```python
from build123d import *

# Parameters (mm, degrees)
ESBO_O1_W                = 126
ESBO_O1_H                = 74
ESBO_O1_W_2              = 120
ESBO_O1_H_2              = 68
RESSALTO_EXTRUS_O1_DEPTH = 60
ESBO_O2_W                = 126
ESBO_O2_H                = 74
ESBO_O2_R                = 2
RESSALTO_EXTRUS_O2_DEPTH = 2
ESBO_O3_W                = 25
ESBO_O3_H                = 25
ESBO_O3_W_2              = 14
ESBO_O3_H_2              = 16
ESBO_O3_W_3              = 10
ESBO_O3_H_3              = 30
CORTE_EXTRUS_O1_DEPTH    = 10
ESBO_O6_W                = 8
ESBO_O6_H                = 40
CORTE_EXTRUS_O2_DEPTH    = 115.214710086
ESBO_O7_W                = 10
ESBO_O7_H                = 30
CORTE_EXTRUS_O3_DEPTH    = 12


with BuildPart() as part:
    # Esboço1 → Ressalto-extrusão1 (new body)
    with BuildSketch(Plane.XY):
        Rectangle(ESBO_O1_W, ESBO_O1_H)
        Rectangle(ESBO_O1_W_2, ESBO_O1_H_2, mode=Mode.SUBTRACT)
    extrude(amount=RESSALTO_EXTRUS_O1_DEPTH)

    # Esboço2 → Ressalto-extrusão2 (add)
    with BuildSketch(Plane(origin=(0, 0, 0), x_dir=(-1, 0, 0), z_dir=(0, 0, -1))):
        Rectangle(ESBO_O2_W, ESBO_O2_H)
        with Locations((-54, -28)):
            Circle(ESBO_O2_R, mode=Mode.SUBTRACT)
        with Locations((54, -28)):
            Circle(ESBO_O2_R, mode=Mode.SUBTRACT)
        with Locations((54, 28)):
            Circle(ESBO_O2_R, mode=Mode.SUBTRACT)
        with Locations((-54, 28)):
            Circle(ESBO_O2_R, mode=Mode.SUBTRACT)
    extrude(amount=RESSALTO_EXTRUS_O2_DEPTH)

    # Esboço3 → Corte-extrusão1 (cut)
    with BuildSketch(Plane(origin=(63, 0, 0), x_dir=(0, 0, -1), z_dir=(1, 0, 0))):
        with Locations((-23.5, 19.5)):
            Rectangle(ESBO_O3_W, ESBO_O3_H)
        with Locations((-7, -15.5)):
            Rectangle(ESBO_O3_W_2, ESBO_O3_H_2)
        with Locations((-45, 0)):
            Rectangle(ESBO_O3_W_3, ESBO_O3_H_3)
    extrude(amount=-CORTE_EXTRUS_O1_DEPTH, mode=Mode.SUBTRACT)

    # Esboço6 → Corte-extrusão2 (cut, through all)
    with BuildSketch(Plane.XZ.offset(37)):
        with Locations((-49, 28)):
            Rectangle(ESBO_O6_W, ESBO_O6_H)
        with Locations((-36, 28)):
            Rectangle(ESBO_O6_W, ESBO_O6_H)
        with Locations((-23, 28)):
            Rectangle(ESBO_O6_W, ESBO_O6_H)
        with Locations((-10, 28)):
            Rectangle(ESBO_O6_W, ESBO_O6_H)
        with Locations((3, 28)):
            Rectangle(ESBO_O6_W, ESBO_O6_H)
        with Locations((16, 28)):
            Rectangle(ESBO_O6_W, ESBO_O6_H)
        with Locations((29, 28)):
            Rectangle(ESBO_O6_W, ESBO_O6_H)
        with Locations((42, 28)):
            Rectangle(ESBO_O6_W, ESBO_O6_H)
    extrude(amount=-CORTE_EXTRUS_O2_DEPTH, mode=Mode.SUBTRACT)

    # Esboço7 → Corte-extrusão3 (cut)
    with BuildSketch(Plane.ZY.offset(63)):
        with Locations((43, 0)):
            Rectangle(ESBO_O7_W, ESBO_O7_H)
        with Locations((23, 0)):
            Rectangle(ESBO_O7_W, ESBO_O7_H)
    extrude(amount=-CORTE_EXTRUS_O3_DEPTH, mode=Mode.SUBTRACT)


solid = part.part
```
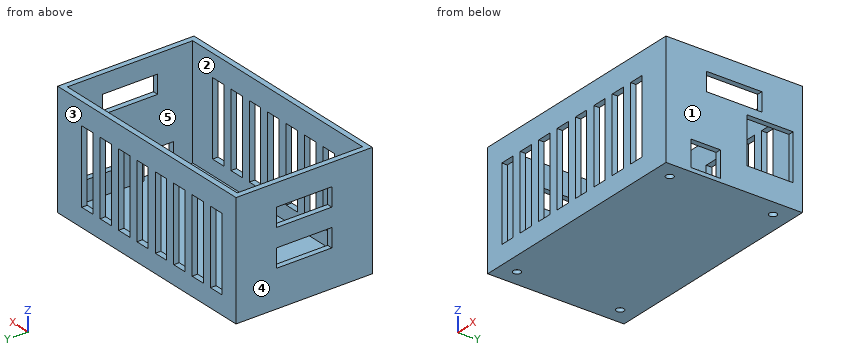
Can you work these out from the model? Positions are in its coordinate system, mm. Face numbers are marked on the shaded views. A direction names the side the tool comes from. Coordinates: 2 decimals unless noted, no trailing zeros. Loops run counter-clockwise (first coordinate to the right, second up) from the corner with the lowest first, then second, coordinate; pieces in that order, holes last. Notation, with made-up numbers: (-37, 39) -> (-17, 39) arc R4 cw to (-17, 43) -> close; hole circle Ø9 at (82.25, -35). An arc over 180 degrees is marked (long way). Put each result on its own line as item: value. Start each with the question number.
Q1. I want a section at D-D (y = -18.5). Write out the boundary of the cut face in (x, z), plus the area to 3 significant figures.
Q2. Thinking about a two-plate mould opening in Y: for the marked faces 3, 4 and 5, which applies, pulls with the +Y half, pulls with the -Y half, needs draft (parallel to the pull), parting line crosses it, or undercut?
Q3. I want a section at A-A (y = 28). Write out the boundary of the cut face in (x, z), plus the area to 3 significant figures.
Q4. I want a section at C-C (x = -22). Write out the boundary of the cut face in (y, z), plus the area to 3 significant figures.
Q5. If I drill on line 1 (Y direction, x = -48.5, z = 3); line 2 (X direction, y = -10.5, z = 51.5); line 3 (Y direction, x = -54, z = -1.15), over which ranges is the centre line in solid material (lowest first)? Write a range as [from, to].
Q6. I want a section at B-B (z = 55). Write out the boundary of the cut face in (x, y), plus the area to 3 significant figures.
Q7. I'm going to push flat-ended pins straight in: P1, Ø12, axis at x = -20, y = -22, coming from the +Z side; P2, Ø8, axis at y = -9, z = 26.5, coming from the -X side. Where does each tip first touch, or does it pass through?
Q8. For the marked faces 1 and 2, which set-ups out of +Z, -Z, +X, -X, +Y, -Y let a thin tool reach every point of the face, with its end or its side?
Taken from the geometry:
1. outline: (-63, -2) -> (63, -2) -> (63, 0) -> (-60, 0) -> (-60, 60) -> (-63, 60) -> close; (60, 14) -> (63, 14) -> (63, 60) -> (60, 60) -> close
1. area: 570 mm2
2. face 3: pulls with the +Y half
2. face 4: needs draft
2. face 5: undercut
3. outline: (-63, -2) -> (-56, -2) -> (-56, 0) -> (-60, 0) -> (-60, 60) -> (-63, 60) -> close; (-52, -2) -> (52, -2) -> (52, 0) -> (-52, 0) -> close; (56, -2) -> (63, -2) -> (63, 11) -> (60, 11) -> (60, 0) -> (56, 0) -> close; (60, 36) -> (63, 36) -> (63, 60) -> (60, 60) -> close
3. area: 521 mm2
4. outline: (-37, -2) -> (37, -2) -> (37, 8) -> (34, 8) -> (34, 0) -> (-34, 0) -> (-34, 8) -> (-37, 8) -> close; (-37, 48) -> (-34, 48) -> (-34, 60) -> (-37, 60) -> close; (34, 48) -> (37, 48) -> (37, 60) -> (34, 60) -> close
4. area: 268 mm2
5. line 1: y = [-37, -34], [34, 37]
5. line 2: x = [-63, -60], [60, 63]
5. line 3: y = [-37, -30], [-26, 26], [30, 37]
6. outline: (-63, -37) -> (63, -37) -> (63, 37) -> (-63, 37) -> close; hole (-60, -34) -> (60, -34) -> (60, 34) -> (-60, 34) -> close
6. area: 1,160 mm2
7. P1: stops at z = 0
7. P2: stops at x = -63
8. face 1: +Z, -Z, +X, +Y, -Y
8. face 2: +Z
